```python
from build123d import *

# Parameters (mm, degrees)
SKETCH1_W           = 30
SKETCH1_H           = 39.485211854
BOSS_EXTRUDE1_DEPTH = 2.5
SKETCH2_W           = 14.50000216
SKETCH2_H           = 24.699998732
CUT_EXTRUDE1_DEPTH  = 37.000350752
CHAMFER2_SIZE       = 3
FILLET5_R           = 3.7
BOSS_EXTRUDE2_DEPTH = 5


with BuildPart() as part:
    # Sketch1 → Boss-Extrude1 (new body)
    with BuildSketch(Plane.XY):
        with Locations((15.000000036, -0.000120634)):
            Rectangle(SKETCH1_W, SKETCH1_H)
    extrude(amount=BOSS_EXTRUDE1_DEPTH)

    # Sketch2 → Cut-Extrude1 (cut, through all)
    with BuildSketch(Plane.XY.offset(2.5)):
        with Locations((13.737600789, -1.949e-06)):
            Rectangle(SKETCH2_W, SKETCH2_H)
    extrude(amount=-CUT_EXTRUDE1_DEPTH, mode=Mode.SUBTRACT)

    # Chamfer2
    # the kernel refuses this chamfer: 3 mm, written as the material it takes off along each edge
    with BuildSketch(Plane(origin=(20.987601869, -12.350001315, 2.5), x_dir=(0, -1, 0), z_dir=(-1, 0, 0)), Plane(origin=(6.487599709, 12.349997417, 2.5), x_dir=(0, 1, 0), z_dir=(1, 0, 0))) as chamfer2_piece_1:
        Polygon((CHAMFER2_SIZE, 0), (0, -CHAMFER2_SIZE), (0, 0), align=None)
    extrude(amount=14.500002159, mode=Mode.SUBTRACT)
    with BuildSketch(Plane(origin=(20.987601869, 12.349997417, 2.5), x_dir=(1, 0, 0), z_dir=(0, -1, 0)), Plane(origin=(6.487599709, -12.350001315, 2.5), x_dir=(-1, 0, 0), z_dir=(0, 1, 0))) as chamfer2_piece_2:
        Polygon((CHAMFER2_SIZE, 0), (0, -CHAMFER2_SIZE), (0, 0), align=None)
    extrude(amount=24.699998732, mode=Mode.SUBTRACT)
    with BuildSketch(Plane(origin=(20.987601869, 12.349997417, 2.5), x_dir=(1, 0, 0), z_dir=(0, -1, 0))) as chamfer2_piece_3a_section:
        Polygon((CHAMFER2_SIZE, 0), (0, -CHAMFER2_SIZE), (0, 0), align=None)
    chamfer2_piece_3a = extrude(amount=32.415047696, mode=Mode.PRIVATE)
    chamfer2_piece_3a = split(chamfer2_piece_3a, bisect_by=Plane(origin=(20.987601869, -12.350001315, 2.5), z_dir=(0, -1, 0)), keep=Keep.TOP, mode=Mode.PRIVATE)
    with BuildSketch(Plane(origin=(28.702650833, -12.350001315, 2.5), x_dir=(0, -1, 0), z_dir=(-1, 0, 0))) as chamfer2_piece_3b_section:
        Polygon((CHAMFER2_SIZE, 0), (0, -CHAMFER2_SIZE), (0, 0), align=None)
    chamfer2_piece_3b = extrude(amount=22.215051123, mode=Mode.PRIVATE)
    chamfer2_piece_3b = split(chamfer2_piece_3b, bisect_by=Plane(origin=(20.987601869, -12.350001315, 2.5), z_dir=(1, 0, 0)), keep=Keep.TOP, mode=Mode.PRIVATE)
    chamfer2_piece_3 = chamfer2_piece_3a & chamfer2_piece_3b
    add(chamfer2_piece_3, mode=Mode.SUBTRACT)
    with BuildSketch(Plane(origin=(20.987601869, -12.350001315, 2.5), x_dir=(0, -1, 0), z_dir=(-1, 0, 0))) as chamfer2_piece_4a_section:
        Polygon((CHAMFER2_SIZE, 0), (0, -CHAMFER2_SIZE), (0, 0), align=None)
    chamfer2_piece_4a = extrude(amount=22.215051123, mode=Mode.PRIVATE)
    chamfer2_piece_4a = split(chamfer2_piece_4a, bisect_by=Plane(origin=(6.487599709, -12.350001315, 2.5), z_dir=(-1, 0, 0)), keep=Keep.TOP, mode=Mode.PRIVATE)
    with BuildSketch(Plane(origin=(6.487599709, -20.065050279, 2.5), x_dir=(-1, 0, 0), z_dir=(0, 1, 0))) as chamfer2_piece_4b_section:
        Polygon((CHAMFER2_SIZE, 0), (0, -CHAMFER2_SIZE), (0, 0), align=None)
    chamfer2_piece_4b = extrude(amount=32.415047696, mode=Mode.PRIVATE)
    chamfer2_piece_4b = split(chamfer2_piece_4b, bisect_by=Plane(origin=(6.487599709, -12.350001315, 2.5), z_dir=(0, -1, 0)), keep=Keep.TOP, mode=Mode.PRIVATE)
    chamfer2_piece_4 = chamfer2_piece_4a & chamfer2_piece_4b
    add(chamfer2_piece_4, mode=Mode.SUBTRACT)
    with BuildSketch(Plane(origin=(6.487599709, 12.349997417, 2.5), x_dir=(0, 1, 0), z_dir=(1, 0, 0))) as chamfer2_piece_5a_section:
        Polygon((CHAMFER2_SIZE, 0), (0, -CHAMFER2_SIZE), (0, 0), align=None)
    chamfer2_piece_5a = extrude(amount=22.215051123, mode=Mode.PRIVATE)
    chamfer2_piece_5a = split(chamfer2_piece_5a, bisect_by=Plane(origin=(20.987601869, 12.349997417, 2.5), z_dir=(1, 0, 0)), keep=Keep.TOP, mode=Mode.PRIVATE)
    with BuildSketch(Plane(origin=(20.987601869, 20.065046381, 2.5), x_dir=(1, 0, 0), z_dir=(0, -1, 0))) as chamfer2_piece_5b_section:
        Polygon((CHAMFER2_SIZE, 0), (0, -CHAMFER2_SIZE), (0, 0), align=None)
    chamfer2_piece_5b = extrude(amount=32.415047696, mode=Mode.PRIVATE)
    chamfer2_piece_5b = split(chamfer2_piece_5b, bisect_by=Plane(origin=(20.987601869, 12.349997417, 2.5), z_dir=(0, 1, 0)), keep=Keep.TOP, mode=Mode.PRIVATE)
    chamfer2_piece_5 = chamfer2_piece_5a & chamfer2_piece_5b
    add(chamfer2_piece_5, mode=Mode.SUBTRACT)
    with BuildSketch(Plane(origin=(-1.227449254, 12.349997417, 2.5), x_dir=(0, 1, 0), z_dir=(1, 0, 0))) as chamfer2_piece_6a_section:
        Polygon((CHAMFER2_SIZE, 0), (0, -CHAMFER2_SIZE), (0, 0), align=None)
    chamfer2_piece_6a = extrude(amount=22.215051123, mode=Mode.PRIVATE)
    chamfer2_piece_6a = split(chamfer2_piece_6a, bisect_by=Plane(origin=(6.487599709, 12.349997417, 2.5), z_dir=(-1, 0, 0)), keep=Keep.TOP, mode=Mode.PRIVATE)
    with BuildSketch(Plane(origin=(6.487599709, -12.350001315, 2.5), x_dir=(-1, 0, 0), z_dir=(0, 1, 0))) as chamfer2_piece_6b_section:
        Polygon((CHAMFER2_SIZE, 0), (0, -CHAMFER2_SIZE), (0, 0), align=None)
    chamfer2_piece_6b = extrude(amount=32.415047696, mode=Mode.PRIVATE)
    chamfer2_piece_6b = split(chamfer2_piece_6b, bisect_by=Plane(origin=(6.487599709, 12.349997417, 2.5), z_dir=(0, 1, 0)), keep=Keep.TOP, mode=Mode.PRIVATE)
    chamfer2_piece_6 = chamfer2_piece_6a & chamfer2_piece_6b
    add(chamfer2_piece_6, mode=Mode.SUBTRACT)

    # Fillet5
    # the kernel refuses this fillet: 3.7 mm, written as the material it takes off along each edge
    with BuildSketch(Plane(origin=(-8.749999964, 19.742485293, 2.5), x_dir=(0, 0, -1), z_dir=(1, 0, 0))) as fillet5_piece_1:
        with BuildLine():
            CenterArc((3.7, -3.5), FILLET5_R, 108.924644416, 71.075355584)
            Line((0, -3.5), (0, 0))
            Line((0, 0), (2.5, 0))
        make_face()
    extrude(amount=47.5, mode=Mode.SUBTRACT)
    with BuildSketch(Plane(origin=(38.750000036, -19.742726561, 2.5), x_dir=(0, 1, 0), z_dir=(-1, 0, 0))) as fillet5_piece_2:
        with BuildLine():
            CenterArc((3.5, 3.7), FILLET5_R, 198.924644416, 71.075355584)
            Line((0, 2.5), (0, 0))
            Line((0, 0), (3.5, 0))
        make_face()
    extrude(amount=47.5, mode=Mode.SUBTRACT)
    with BuildSketch(Plane(origin=(3.6e-08, -28.492726561, 2.5), x_dir=(1, 0, 0), z_dir=(0, 1, 0)), Plane(origin=(30.000000036, 28.492485293, 2.5), x_dir=(-1, 0, 0), z_dir=(0, -1, 0))) as fillet5_piece_3:
        with BuildLine():
            CenterArc((3.5, 3.7), FILLET5_R, 198.924644416, 71.075355584)
            Line((0, 2.5), (0, 0))
            Line((0, 0), (3.5, 0))
        make_face()
    extrude(amount=56.985211855, mode=Mode.SUBTRACT)

    # Sketch5 → Boss-Extrude2 (add)
    with BuildSketch(Plane(origin=(0, 0, 0), x_dir=(-1, 0, 0), z_dir=(0, 0, -1))):
        Polygon((-3.6e-08, -19.742726561), (-5.000000036, -19.742726561), (-5.000000036, -17.242726561), (-2.5, -17.242726561), (-2.5, -14.742726561), (0, -14.742726561), align=None)
        Polygon((-2.499996996, 17.242720698), (-4.999997021, 17.242721136), (-4.999996584, 19.742721136), (3.416e-06, 19.742720261), (2.578e-06, 14.742720261), (-2.499997422, 14.742720698), align=None)
    extrude(amount=BOSS_EXTRUDE2_DEPTH)


solid = part.part
```
Work out the finished part from the listing and answer in its coordinate system (mm). A direction names the side the tool comes from. Round coordinates to 2 decimals unless told otherwise and drop trailing zeros. Write each loop counter-clockwise with the first axis right and the second up, starting at its lowest first coordinate (ties: lowest second). Pieces come first, ordered by that corner, then holes.
1) A cutting plane is placed at D-D on x = 25.5. Determine the outline of the cut face in (y, z), and give its area (3 significant figures).
2) Consider probe 1 along Y at (x, z) = (4.5, -4); probe 2 along Z at (x, y) = (18, 16.5); probe 3 along Y at (x, z) = (21, 0.75). Determine where each line is inside the solid, lowest interval first.
3) Determine the mould class of faces 1 (the face through (0, -17, -2)), 2 (the face through (25, 0, 0)), 3 (the face through (13.59, 14.12, 1.27)) for opening direction X: pulls with the +X half, pulls with the -X half, needs draft (parallel to the pull), parting line crosses it, or undercut.
4) Which of the six approach directions +Z, -Z, +X, -X, +Y, -Y give full straight-line access (tool end or side, diameter ignored) to faces 4 (the face through (13.88, -14.12, 1.27)), 5 (the face through (4, -17.243, -2)), 6 (the face through (1, -14.743, -2)), 7 (the face through (5, 18, -2)), 8 (the face through (1.32, -0.28, 1.79))?
5) Flat-ended cylindrical pins translate along their axes: P1, Ø3, axis at y = 18.5, z = -3.5, coming from the +X side; P2, Ø3, axis at y = -13.5, z = -0.5, coming from the +X side; P3, Ø4, axis at y = -3, z = 1, coming from the -X side. Find the tip coordinate at first contact, or state that the pin passes through.
6) A cutting plane is placed at C-C on x = 6.5. Determine the outline of the cut face in (y, z).
7) A cutting plane is placed at A-A on y = -6. Determine the outline of the cut face in (x, z), and give its area (3 significant figures).
8) A cutting plane is placed at B-B on z = -0.75. Determine the outline of the cut face in (x, y).
Entries:
1. outline: (-19.74, 0) - (19.74, 0) arc R3.7 ccw to (16.24, 2.5) - (-16.24, 2.5) arc R3.7 ccw to start
1. area: 94.0 mm2
2. probe 1: y = -19.74 to -17.24, 17.24 to 19.74
2. probe 2: z = 0 to 2.49
2. probe 3: y = -19.39 to -13.6, 13.6 to 19.39
3. face 1: pulls with the -X half
3. face 2: needs draft
3. face 3: undercut
4. face 4: +Z
4. face 5: -Z, +X
4. face 6: -Z, +X, -X
4. face 7: -Z, +X, +Y, -Y
4. face 8: +Z, -X, +Y, -Y
5. P1: stops at x = 5
5. P2: stops at x = 30
5. P3: stops at x = 0
6. outline: (-19.74, 0) - (-12.85, 0) - (-15.35, 2.5) - (-16.24, 2.5) arc R3.7 ccw to start; (12.85, 0) - (19.74, 0) arc R3.7 ccw to (16.24, 2.5) - (15.35, 2.5) - close
7. outline: (0, 0) - (5.99, 0) - (3.49, 2.5) arc R3.7 ccw to start; (21.49, 0) - (30, 0) arc R3.7 ccw to (26.5, 2.5) - (23.99, 2.5) - close
7. area: 25.3 mm2
8. outline: (0, -19.74) - (5, -19.74) - (5, -17.24) - (2.5, -17.24) - (2.5, -14.74) - (0, -14.74) - close; (0, 14.74) - (2.5, 14.74) - (2.5, 17.24) - (5, 17.24) - (5, 19.74) - (0, 19.74) - close
